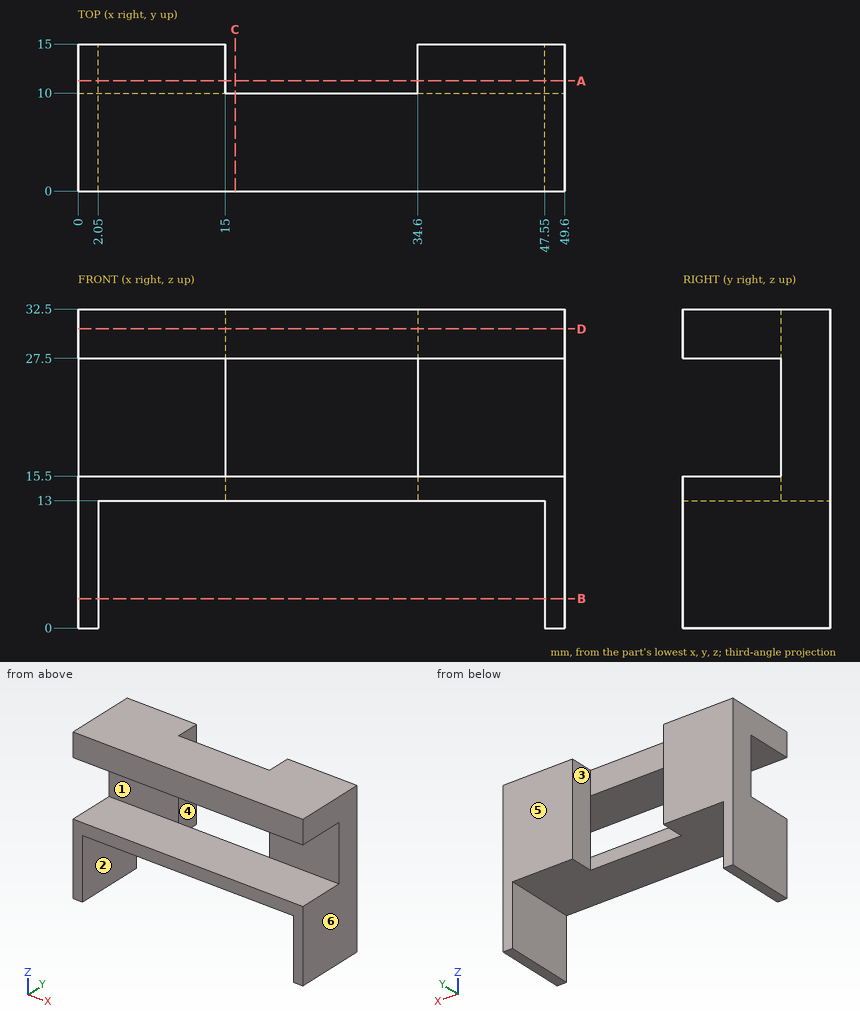
Part print with two shaded views. Sizes in mm from the minimum x, y, z corner. A direction names the side the tool comes from. Give positions to 0.01 mm unless a question says otherwise; leave off trailing zeros. Order: outer loops, then holes, each group sorted by start corner. A loop starts at its lowest first (then second) coordinate and runs counter-clockwise, first axis right, second up. Notation, with made-up numbers: (-36.75, -22) - (-22.75, -22) arc R30 ccw to (-22.75, 15) - close; hole circle Ø7 at (49.25, 7.5). An arc over 180 degrees is marked (long way). Write each question's results on one line, items separated by ' | '.
1. Saw through at A-A on y = 11.25. List the corners of the cut face in (x, z).
Calculated:
outline: (0, 0) - (2.05, 0) - (2.05, 13) - (15, 13) - (15, 32.5) - (0, 32.5) - close; (34.6, 13) - (47.55, 13) - (47.55, 0) - (49.6, 0) - (49.6, 32.5) - (34.6, 32.5) - close
2. Pin check, flat tips, straight feed: pin 1 (2 mm diameter, centred on x = 22, z = 14.5, fed in from +Y); pin 2 (9.5 mm diameter, centred on x = 39, z = 20.5, fed in from -Y); pin 3 (5 mm diameter, centred on x = 44.5, y = 10.5, fed in from -Z); pin 4 (4 mm diameter, centred on y = 4, z = 19, fed in from -X). Stop position of each tip, or through.
Calculated:
pin 1: stops at y = 10 | pin 2: stops at y = 10 | pin 3: stops at z = 13 | pin 4: passes through
3. Saw through at D-D on z = 30.5. List the corners of the cut face in (x, y), and give its area (3 significant figures).
Calculated:
outline: (0, 0) - (49.6, 0) - (49.6, 15) - (34.6, 15) - (34.6, 10) - (15, 10) - (15, 15) - (0, 15) - close | area: 646 mm2
4. Pull direction X, two halves, no side cores. Call the marked faces 4, 5 and 6: released by +X, released by -X, zero draft, split by the parting line, or undercut.
Calculated:
face 4: undercut | face 5: zero draft | face 6: released by +X
5. Saw through at B-B on z = 3. List the corners of the cut face in (x, y).
Calculated:
outline: (0, 0) - (2.05, 0) - (2.05, 15) - (0, 15) - close; (47.55, 0) - (49.6, 0) - (49.6, 15) - (47.55, 15) - close
6. Probe L1, parallel to X at y = 6.75, z = 7; L2, parallel to Z at x = 41, y = 5.5; L3, parallel to X at y = 10.75, z = 25.5. List the from-to ranges inside material, lowest first. Write a range as from..to.
Calculated:
L1: x = 0..2.05, 47.55..49.6 | L2: z = 13..15.5, 27.5..32.5 | L3: x = 0..15, 34.6..49.6
7. 3-axis set-ups, long thin cutter, end or side, ignore diameter. For the marked faces 1, 2 and 3: which of +Z, -Z, +X, -X, +Y, -Y reach the whole face in a straight line?
Calculated:
face 1: +X, -X, -Y | face 2: -Z, +Y, -Y | face 3: +Z, -Z, +Y
8. Saw through at C-C on x = 16. List the corners of the cut face in (y, z).
Calculated:
outline: (0, 13) - (10, 13) - (10, 15.5) - (0, 15.5) - close; (0, 27.5) - (10, 27.5) - (10, 32.5) - (0, 32.5) - close
